Geometry check sheet. Reference: the model listing, model coordinates, mm. A direction names the side the tool comes from. Round coordinates to 2 decimals unless told otherwise and drop trailing zeros. Order: outer loops, then holes, each group sorted by start corner. A loop starts at its lowest first (then second) coordinate and runs counter-clockwise, first axis right, second up. Notation, with made-up numbers: (-6.5, 9.5) - (30.5, 9.5) arc R33 cw to (30.5, 40.5) - close; hole circle Ø5 at (73.25, 84.5). An arc over 180 degrees is marked (long way). Use a Markdown table: item, result. Add a question column.
(1) Thickness scan on line 1 along Z through (x, y) = (10, -4); line 2 along Z through (x, y) = (29, 11); line 3 along Z through (x, y) = (27.5, -16.5). Record the ranges inside material, lowest first. Write a range as [from, to].
(2) Section check A-A on z = 23. Record the boundary of the cut face in (x, y).
(3) Mould release check, pull along Z, two halves, no side actions. Record for faces 1 (the face through (21, 15, 3)), 2 (the face through (13, -24, 7)), 3 (the face through (12.889, -6.872, 53.572)), 4 (the face through (21, 15, 51)): released by +Z, released by -Z, zero draft, split by the parting line, or undercut.
(4) Access from +Z, -Z, +X, -X, +Y, -Y to the whole of each face (thin tool, end or side, straight path). Record for faces 5 (the face through (35.46, 11.13, 53.74)), 6 (the face through (17.567, -17, 8)), 7 (the face through (0, -1, 27)).
(5) Section check B-B on y = -20. Record the boundary of the cut face in (x, z), then the cut area to 3 significant figures.
(6) Section check C-C on z = 11. Record the boundary of the cut face in (x, y), then the cut area to 3 significant figures.
(7) Gauge pin test, flat ends, axial feed: P1, Ø12, axis at y = -5, z = 12, coming from the +X side; P2, Ø3, axis at x = 12, y = -16.5, coming from the +Z side; P3, Ø4.5, axis at x = 16, y = 17.5, coming from the +Z side; P4, Ø6.5, axis at y = -4, z = 7, coming from the -X side. Record the tip position at first contact, or that the pin passes through.
```python
from build123d import *

# Parameters (mm, degrees)
F1_DEPTH      = 54
F2_W          = 28
F2_H          = 48
F3_DEPTH      = 50
F4_W          = 36.3328976004
F4_H          = 48
F5_DEPTH      = 3
F6_W          = 5.7282032303
F6_H          = 48
F7_DEPTH      = 20
F9_DEPTH      = 2
F11_DEPTH     = 2
F13_DEPTH     = 40
F15_DEPTH     = 13
F16_R         = 2.05
F17_DEPTH     = 25
F18_T1_DEPTH  = 46.8928601954
F18_T3_DEPTH  = 61.5
F18_T5_DEPTH  = 6.8839745962
F18_T7_DEPTH  = 30.1666666667
F18_T9_DEPTH  = 56.0044427996
F18_T11_DEPTH = 35.2128129211
F18_T13_DEPTH = 51
F18_T15_DEPTH = 16.667359312
F18_T17_DEPTH = 46.8928601954
F18_T19_DEPTH = 34.6711094662
F18_T24_DEPTH = 1.5
F18_T30_DEPTH = 1.5
F18_T36_DEPTH = 23.6658075373


# Not quite as in the source:
# - a fillet or chamfer that OpenCascade refuses, or shapes differently, is made with other operations: its cross-section is extruded or revolved along the edge and cut away or added


with BuildPart() as f1:
    # F0 (on Top) → F1 (new body)
    with BuildSketch(Plane.XY):
        Polygon((0, -1.5), (0, 0), (8.4, 0), (8.4, -24), (36.1128129211, -24), (36.1128129211, 24.5044427996), (8.4, 8.5044427996), (-2, 2.5), (-2, -1.5), align=None)
    extrude(amount=F1_DEPTH)

    # F2 (on face) → F3 (cut)
    with BuildSketch(Plane(origin=(-1.5825317547, 2.7410254038, 0), x_dir=(-0.8660254038, -0.5, 0), z_dir=(-0.5, 0.8660254038, 0))):
        with Locations((-25.5268347916, 27)):
            Rectangle(F2_W, F2_H)
    extrude(amount=-F3_DEPTH, mode=Mode.SUBTRACT)

    # F4 (on face) → F5 (cut)
    with BuildSketch(Plane(origin=(9.9825317547, 5.7634173958, 0), x_dir=(-0.5, 0.8660254038, 0), z_dir=(0.8660254038, 0.5, 0))):
        with Locations((-16.2013852907, 27)):
            Rectangle(F4_W, F4_H)
    extrude(amount=-F5_DEPTH, mode=Mode.SUBTRACT)

    # F6 (on face) → F7 (cut)
    with BuildSketch(Plane(origin=(34.2312430607, 19.7634173958, 0), x_dir=(0.5, -0.8660254038, 0), z_dir=(-0.8660254038, -0.5, 0))):
        with Locations((0.8990381057, 27)):
            Rectangle(F6_W, F6_H)
    extrude(amount=-F7_DEPTH, mode=Mode.SUBTRACT)

    # F8 (on face) → F9 (cut)
    with BuildSketch(Plane(origin=(0, 0, 51), x_dir=(1, 0, 0), z_dir=(0, 0, -1))):
        Polygon((36.1128129211, -23.1188021535), (36.1128129211, 24), (23.7023471851, 24), (6.4019237886, -5.965212315), align=None)
    extrude(amount=-F9_DEPTH, mode=Mode.SUBTRACT)

    # F10 (on face) → F11 (cut)
    with BuildSketch(Plane.XY.offset(3)):
        Polygon((36.1128129211, 23.1188021535), (6.4019237886, 5.965212315), (23.7023471851, -24), (36.1128129211, -24), align=None)
    extrude(amount=-F11_DEPTH, mode=Mode.SUBTRACT)

    # F12 (on face) → F13 (cut)
    with BuildSketch(Plane.XY.offset(54)):
        Polygon((16.4829037687, -14), (8.4, 0), (8.4, -24), (36.1128129211, -24), (36.1128129211, -2.6666666667), align=None)
    extrude(amount=-F13_DEPTH, mode=Mode.SUBTRACT)

    # F14 (on face) → F15 (cut)
    with BuildSketch(Plane.XY.offset(14)):
        Polygon((23.7023471851, -24), (17.567359312, -13.3738893001), (17.567359312, -24), align=None)
    extrude(amount=-F15_DEPTH, mode=Mode.SUBTRACT)

    # F16 (on face) → F17 (cut)
    with BuildSketch(Plane(origin=(8.4, 0, 0), x_dir=(0, -1, 0), z_dir=(-1, 0, 0))):
        with Locations((20, 7)):
            Circle(F16_R)
        with Locations((4, 7)):
            Circle(F16_R)
    extrude(amount=-F17_DEPTH, mode=Mode.SUBTRACT)

    # F18: fillet of radius 1.5 on 12 edges, made by hand

    # F18_s2 → F18_t1 (cut)
    with BuildSketch(Plane(origin=(0.3325317547, 0.1919872981, 0), x_dir=(0, 0, 1), z_dir=(0.8660254038, 0.5, 0))):
        with BuildLine():
            ThreePointArc((54, -1.6650635095), (53.5606601718, -2.7257236812), (52.5, -3.1650635095))
            Line((52.5, -3.1650635095), (54, -3.1650635095))
            Line((54, -3.1650635095), (54, -1.6650635095))
        make_face()
    extrude(amount=F18_T1_DEPTH, mode=Mode.SUBTRACT)

    # F18_s4 → F18_t3 (cut)
    with BuildSketch(Plane.XY.offset(-3.75)):
        with BuildLine():
            ThreePointArc((-0.5, -1.5), (-1.5606601718, -1.0606601718), (-2, 0))
            Line((-2, 0), (-2, -1.5))
            Line((-2, -1.5), (-0.5, -1.5))
        make_face()
    extrude(amount=F18_T3_DEPTH, mode=Mode.SUBTRACT)

    # F18_s6 → F18_t5 (cut)
    with BuildSketch(Plane.XZ.offset(-1.6339745962)):
        with BuildLine():
            ThreePointArc((-0.5, 54), (-1.5606601718, 53.5606601718), (-2, 52.5))
            Line((-2, 52.5), (-2, 54))
            Line((-2, 54), (-0.5, 54))
        make_face()
        with BuildLine():
            ThreePointArc((-0.5, 0), (-1.5606601718, 0.4393398282), (-2, 1.5))
            Line((-2, 1.5), (-2, 0))
            Line((-2, 0), (-0.5, 0))
        make_face()
    extrude(amount=F18_T5_DEPTH, mode=Mode.SUBTRACT)

    # F18_s8 → F18_t7 (cut)
    with BuildSketch(Plane(origin=(29.1775044166, 16.8456400292, 0), x_dir=(0, 0, 1), z_dir=(-0.8660254038, -0.5, 0))):
        with BuildLine():
            ThreePointArc((54, -18.8658075373), (53.5606601718, -19.9264677091), (52.5, -20.3658075373))
            Line((52.5, -20.3658075373), (54, -20.3658075373))
            Line((54, -20.3658075373), (54, -18.8658075373))
        make_face()
    extrude(amount=F18_T7_DEPTH, mode=Mode.SUBTRACT)

    # F18_s10 → F18_t9 (cut)
    with BuildSketch(Plane.XZ.offset(-28.2544427996)):
        with BuildLine():
            ThreePointArc((34.6128129211, 0), (35.6734730929, 0.4393398282), (36.1128129211, 1.5))
            Line((36.1128129211, 1.5), (36.1128129211, 0))
            Line((36.1128129211, 0), (34.6128129211, 0))
        make_face()
    extrude(amount=F18_T9_DEPTH, mode=Mode.SUBTRACT)

    # F18_s12 → F18_t11 (cut)
    with BuildSketch(Plane.YZ.offset(4.65)):
        with BuildLine():
            ThreePointArc((-22.5, 0), (-23.5606601718, 0.4393398282), (-24, 1.5))
            Line((-24, 1.5), (-24, 0))
            Line((-24, 0), (-22.5, 0))
        make_face()
    extrude(amount=F18_T11_DEPTH, mode=Mode.SUBTRACT)

    # F18_s14 → F18_t13 (cut)
    with BuildSketch(Plane.XY.offset(1.5)):
        with BuildLine():
            ThreePointArc((-2, 1.6339745962), (-1.7990381057, 2.3839745962), (-1.25, 2.9330127019))
            Line((-1.25, 2.9330127019), (-2, 2.5))
            Line((-2, 2.5), (-2, 1.6339745962))
        make_face()
    extrude(amount=F18_T13_DEPTH, mode=Mode.SUBTRACT)

    # F18_s16 → F18_t15 (cut)
    with BuildSketch(Plane.YZ.offset(4.65)):
        with BuildLine():
            ThreePointArc((-24, 12.5), (-23.5606601718, 13.5606601718), (-22.5, 14))
            Line((-22.5, 14), (-24, 14))
            Line((-24, 14), (-24, 12.5))
        make_face()
    extrude(amount=F18_T15_DEPTH, mode=Mode.SUBTRACT)

    # F18_s18 → F18_t17 (cut)
    with BuildSketch(Plane(origin=(40.94293994, 23.6384173958, 0), x_dir=(0, 0, 1), z_dir=(-0.8660254038, -0.5, 0))):
        with BuildLine():
            ThreePointArc((0, 1.6650635095), (0.4393398282, 2.7257236812), (1.5, 3.1650635095))
            Line((1.5, 3.1650635095), (0, 3.1650635095))
            Line((0, 3.1650635095), (0, 1.6650635095))
        make_face()
    extrude(amount=F18_T17_DEPTH, mode=Mode.SUBTRACT)

    # F18_s20 → F18_t19 (cut)
    with BuildSketch(Plane.XZ.offset(-28.2544427996)):
        with BuildLine():
            ThreePointArc((34.6128129211, 54), (35.6734730929, 53.5606601718), (36.1128129211, 52.5))
            Line((36.1128129211, 52.5), (36.1128129211, 54))
            Line((36.1128129211, 54), (34.6128129211, 54))
        make_face()
    extrude(amount=F18_T19_DEPTH, mode=Mode.SUBTRACT)


with BuildPart() as f18_tool22:
    # F18_s23 → F18_t24 (new body)
    with BuildSketch(Plane.XY.offset(52.5)):
        Polygon((-0.5, 1.6339745962), (-2, 1.6339745962), (-2, 2.5), (-1.25, 2.9330127019), align=None)
    extrude(amount=F18_T24_DEPTH)

    # F18_s25 → F18_t26 (revolve, cut)
    with BuildSketch(Plane(origin=(-0.5, 1.6339745962, 52.5), x_dir=(0.8660254038, -0.5, 0), z_dir=(-0.5, -0.8660254038, 0))):
        with BuildLine():
            ThreePointArc((0, -1.5), (1.5, 0), (0, 1.5))
            Line((0, 1.5), (0, -1.5))
        make_face()
    revolve(axis=Axis((-0.5, 1.6339745962, 52.5), (0, 0, 1)), mode=Mode.SUBTRACT)


with BuildPart() as f1_1:
    add(f1.part)

    # F18_t21: cut F18_tool22
    add(f18_tool22.part, mode=Mode.SUBTRACT)


with BuildPart() as f18_tool28:
    # F18_s29 → F18_t30 (new body)
    with BuildSketch(Plane.XY.offset(1.5)):
        Polygon((-0.5, 1.6339745962), (-2, 1.6339745962), (-2, 2.5), (-1.25, 2.9330127019), align=None)
    extrude(amount=-F18_T30_DEPTH)

    # F18_s31 → F18_t32 (revolve, cut)
    with BuildSketch(Plane(origin=(-0.5, 1.6339745962, 1.5), x_dir=(0.8660254038, -0.5, 0), z_dir=(0.5, 0.8660254038, 0))):
        with BuildLine():
            ThreePointArc((0, -1.5), (1.5, 0), (0, 1.5))
            Line((0, 1.5), (0, -1.5))
        make_face()
    revolve(axis=Axis((-0.5, 1.6339745962, 1.5), (0, 0, -1)), mode=Mode.SUBTRACT)


with BuildPart() as f1_2:
    add(f1_1.part)

    # F18_t27: cut F18_tool28
    add(f18_tool28.part, mode=Mode.SUBTRACT)


with BuildPart() as f18_tool34:
    # F18_s35 → F18_t36 (new body)
    with BuildSketch(Plane(origin=(12.0579037687, -20.8849019601, 0), x_dir=(0, 0, 1), z_dir=(-0.5, 0.8660254038, 0))):
        with BuildLine():
            ThreePointArc((54, 8.7746133918), (53.5606601718, 7.71395322), (52.5, 7.2746133918))
            Line((52.5, 7.2746133918), (54, 7.2746133918))
            Line((54, 7.2746133918), (54, 8.7746133918))
        make_face()
    extrude(amount=F18_T36_DEPTH)

    split(bisect_by=Plane.XZ, keep=Keep.TOP)


with BuildPart() as f1_3:
    add(f1_2.part)

    # F18_t33: cut F18_tool34
    add(f18_tool34.part, mode=Mode.SUBTRACT)


solid = f1_3.part
```
Check sheet entries:
| question | item | result |
|---|---|---|
| 1 | line 1 | z = [0, 4.95], [9.05, 14] |
| 1 | line 2 | z = [0, 1], [53, 54] |
| 1 | line 3 | z = [0, 1] |
| 2 | outline | (-2, 0) arc R1.5 ccw to (-0.5, -1.5) - (0, -1.5) - (0, 0) - (8.4, 0) - (16.48, -14) - (17.57, -13.37) - (6.4, 5.97) - (9, 7.47) - (8.4, 8.5) - (-1.25, 2.93) arc R1.5 ccw to (-2, 1.63) - close; (32.65, 22.5) - (33.25, 21.47) - (36.11, 23.12) - (36.11, 24.5) - close |
| 3 | face 1 | undercut |
| 3 | face 2 | zero draft |
| 3 | face 3 | released by +Z |
| 3 | face 4 | undercut |
| 4 | face 5 | +Z, +X, +Y, -Y |
| 4 | face 6 | +Z, +X, -Y |
| 4 | face 7 | +Z, -Z, -Y |
| 5 | outline | (8.4, 0) - (34.61, 0) arc R1.5 ccw to (36.03, 1) - (17.57, 1) - (17.57, 4.95) - (8.4, 4.95) - close; (8.4, 9.05) - (17.57, 9.05) - (17.57, 14) - (8.4, 14) - close |
| 5 | area | 109 mm2 |
| 6 | outline | (-2, 0) arc R1.5 ccw to (-0.5, -1.5) - (0, -1.5) - (0, 0) - (8.4, 0) - (8.4, -24) - (17.57, -24) - (17.57, -13.37) - (6.4, 5.97) - (9, 7.47) - (8.4, 8.5) - (-1.25, 2.93) arc R1.5 ccw to (-2, 1.63) - close; (32.65, 22.5) - (33.25, 21.47) - (36.11, 23.12) - (36.11, 24.5) - close |
| 6 | area | 230 mm2 |
| 7 | P1 | stops at x = 16.2 |
| 7 | P2 | stops at z = 14 |
| 7 | P3 | passes through |
| 7 | P4 | stops at x = -1.8 |
